from build123d import *

# Parameters (mm, degrees)
SKETCH1_W              = 10
SKETCH1_H              = 18
BOSS_EXTRUDE1_DEPTH    = 7
SKETCH2_W              = 10
SKETCH2_H              = 6
CUT_EXTRUDE1_DEPTH     = 0.5
M2_5_CLEARANCE_HOLE1_D = 2.7
SKETCH5_W              = 10
SKETCH5_H              = 6
CUT_EXTRUDE2_DEPTH     = 3
M2_5_CLEARANCE_HOLE2_D = 2.7


with BuildPart() as part:
    # Sketch1 → Boss-Extrude1 (new body)
    with BuildSketch(Plane(origin=(0, 0, 0), x_dir=(1, 0, 0), z_dir=(0, 1, 0))):
        Rectangle(SKETCH1_W, SKETCH1_H)
    extrude(amount=BOSS_EXTRUDE1_DEPTH)

    # Sketch2 → Cut-Extrude1 (cut)
    with BuildSketch(Plane(origin=(0, 7, 0), x_dir=(1, 0, 0), z_dir=(0, 1, 0))):
        with Locations((0, 6)):
            Rectangle(SKETCH2_W, SKETCH2_H)
    extrude(amount=-CUT_EXTRUDE1_DEPTH, mode=Mode.SUBTRACT)

    # M2.5 Clearance Hole1 (through all)
    with Locations(Plane(origin=(0, 7, 0), x_dir=(1, 0, 0), z_dir=(0, 1, 0))):
        with Locations((-2.5, -6.5), (2.5, 0.5)):
            Hole(M2_5_CLEARANCE_HOLE1_D / 2)

    # Sketch5 → Cut-Extrude2 (cut)
    with BuildSketch(Plane.XZ):
        with Locations((0, -6)):
            Rectangle(SKETCH5_W, SKETCH5_H)
    extrude(amount=-CUT_EXTRUDE2_DEPTH, mode=Mode.SUBTRACT)

    # M2.5 Clearance Hole2 (through all)
    with Locations(Plane(origin=(0, 3, 0), x_dir=(-1, 0, 0), z_dir=(0, -1, 0))):
        with Locations((-2.5, 6), (2.5, 6)):
            Hole(M2_5_CLEARANCE_HOLE2_D / 2)


solid = part.part
Could you check a few things on this model? Use its own coordinates, in mm. A direction names the side the tool comes from. Give positions to 0.01 mm unless a question says otherwise; leave off trailing zeros. Order: outer loops, then holes, each group sorted by start corner. A loop starts at its lowest first (then second) coordinate and runs counter-clockwise, first axis right, second up.
Item 1: I need wall thicknesses on line 1 (X direction, y = 4.35, z = -6); line 2 (Z direction, x = 2.5, y = 4.75); line 3 (Z direction, x = -2.5, y = 6). Which ranges of each line are inside material? Lowest first, please.
Item 2: If we section it at A-A, the plane x = 2.5: Write out the boundary of the cut face in (y, z).
Item 3: I'm going to push flat-ended pins straight in: pin 1 (2 mm diameter, centred on x = 2.5, z = -6, fed in from +Y); pin 2 (2.5 mm diameter, centred on x = -2, y = 1.5, fed in from -Z); pin 3 (1.8 mm diameter, centred on x = 1, z = -6, fed in from -Y); pin 4 (5 mm diameter, centred on x = -1.5, z = -6, fed in from +Y). Where does each tip first touch, or does it pass through?
Item 4: If we section it at C-C, the plane z = 6.5: Write out the boundary of the cut face in (x, y).
Item 5: If we mould it in two halves opening along X, with no side actions, what happens to faces 4 (the face through (-2.324, 3.451, 5.161)), 5 (the face through (-5, 3, 2)), 6 (the face through (0, 7, 3)), 7 (the face through (5, 3, 2))? For each: pulls with the +X half, pulls with the -X half, needs draft (parallel to the pull), parting line crosses it, or undercut.
Item 6: If we section it at B-B, the plane y = 3.25: Write out the boundary of the cut face in (x, z), plus the area to 3 significant figures.
Item 7: If we section it at D-D, the plane z = -6: Write out the boundary of the cut face in (x, y).
Item 8: For faces 1 (the face through (0, 6.5, -6)), 2 (the face through (0, 1, -3)), 3 (the face through (2.324, 4.774, -7.339)), which set-ups out of +Z, -Z, +X, -X, +Y, -Y let a thin tool reach every point of the face, with its end or its side?
Values:
1. line 1: x = -5 to -3.85, -1.15 to 1.15, 3.85 to 5
1. line 2: z = -9 to -7.35, -4.65 to -1.85, 0.85 to 9
1. line 3: z = -9 to -7.35, -4.65 to 5.15, 7.85 to 9
2. outline: (0, -3) - (3, -3) - (3, -4.65) - (6.5, -4.65) - (6.5, -3) - (7, -3) - (7, -1.85) - (0, -1.85) - close; (0, 0.85) - (7, 0.85) - (7, 9) - (0, 9) - close; (3, -9) - (6.5, -9) - (6.5, -7.35) - (3, -7.35) - close
3. pin 1: passes through
3. pin 2: stops at z = -3
3. pin 3: stops at y = 3
3. pin 4: stops at y = 6.5
4. outline: (-5, 0) - (-3.85, 0) - (-3.85, 7) - (-5, 7) - close; (-1.15, 0) - (5, 0) - (5, 7) - (-1.15, 7) - close
5. face 4: undercut
5. face 5: pulls with the -X half
5. face 6: needs draft
5. face 7: pulls with the +X half
6. outline: (-5, -9) - (5, -9) - (5, 9) - (-5, 9) - close; hole circle Ø2.7 at (-2.5, -6); hole circle Ø2.7 at (-2.5, 6.5); hole circle Ø2.7 at (2.5, -6); hole circle Ø2.7 at (2.5, -0.5)
6. area: 157 mm2
7. outline: (-5, 3) - (-3.85, 3) - (-3.85, 6.5) - (-5, 6.5) - close; (-1.15, 3) - (1.15, 3) - (1.15, 6.5) - (-1.15, 6.5) - close; (3.85, 3) - (5, 3) - (5, 6.5) - (3.85, 6.5) - close
8. face 1: -Z, +X, -X, +Y
8. face 2: -Z, +X, -X, -Y
8. face 3: +Y, -Y
